Job drawing, mm, ordinate dimensions from the low corner. One solid piece. Coordinates: 2 decimals unless noted, no trailing zeros. Write each loop counter-clockwise with the first axis right and the second up, starting at its lowest first coordinate (ties: lowest second). Pieces come first, ordered by that corner, then holes.
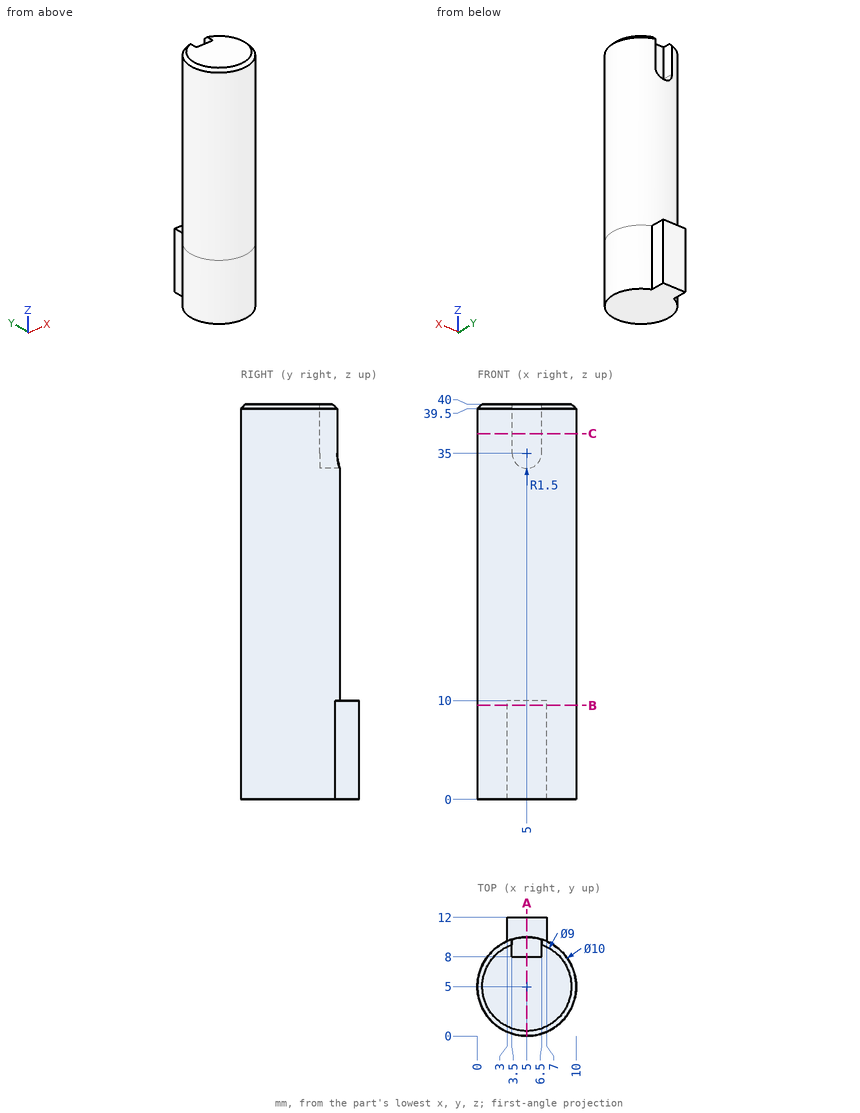
1. Probe line 1 along Y through (x, z) = (5.25, 23); line 2 along X through (y, z) = (9, 37.5); line 3 along Y through (x, z) = (1.25, 4.5). List the from-to ranges inside material, lowest first.
Computed values:
line 1: y = 0.01 to 9.99
line 2: x = 2 to 3.5, 6.5 to 8
line 3: y = 1.69 to 8.31
2. Saw through at A-A on x = 5. List the corners of the cut face in (y, z), plus the area to 3 significant figures.
Computed values:
outline: (0, 0) - (12, 0) - (12, 10) - (10, 10) - (10, 33.5) - (8, 33.5) - (8, 40) - (0.5, 40) - (0, 39.5) - close
area: 407 mm2
3. Flat gauge pins, fed straight in: pin 1 (1.5 mm diameter, centred on y = 3, z = 14.5, fed in from -X); pin 2 (2.5 mm diameter, centred on x = 5, z = 37.5, fed in from +Y); pin 3 (1.9 mm diameter, centred on y = 11, z = 3.5, fed in from -X). Where does each tip first touch, or does it go through?
Computed values:
pin 1: stops at x = 0.16
pin 2: stops at y = 8
pin 3: stops at x = 3
4. Saw through at C-C on z = 37. List the corners of the cut face in (x, y), plus the area to 3 significant figures.
Computed values:
outline: (3.5, 8) - (3.5, 9.77) arc R5 ccw (long way) to (6.5, 9.77) - (6.5, 8) - close
area: 72.8 mm2
5. Saw through at B-B on z = 9.5. List the corners of the cut face in (x, y).
Computed values:
outline: (3, 9.58) arc R5 ccw (long way) to (7, 9.58) - (7, 12) - (3, 12) - close
